Build history of the part. All positions in model axes, mm. A direction names the side the tool comes from. Round coordinates to 2 decimals unless told otherwise and drop trailing zeros. Loops run counter-clockwise (first coordinate to the right, second up) from the corner with the lowest first, then second, coordinate; pieces in that order, holes last. Notation, with made-up numbers: (-17.5, 88.25) - (5.5, 88.25) arc R28 cw to (5.5, 127.25) - close; hole circle Ø1 at (-16.75, 66). An arc over 180 degrees is marked (long way). Put each result on its own line as item: value. Start each with the question number.
Autodesk Inventor part; units mm, degrees
ref_plane "YZ Plane" through (0, 0, 0) normal (1, 0, 0) x (0, 1, 0)
ref_plane "XZ Plane" through (0, 0, 0) normal (0, 1, 0) x (-1, 0, 0)
ref_plane "XY Plane" through (0, 0, 0) normal (0, 0, 1) x (1, 0, 0)
sketch "Sketch1" plane through (0, 0, 0) normal (0, 0, 1) x (1, 0, 0)
  circle A0 centre (0, 0) radius 47.625
  dimension "d0" = 95.25
extrude "Extrusion1" add sketch "Sketch1" along normal blind 3.175
sketch "Sketch3" plane through (0, 0, 3.175) normal (0, 0, 1) x (1, 0, 0)
  line L0 (1.27, 9.525) -> (20.32, 9.525)
  line L1 (20.32, 9.525) -> (20.32, 0)
  line L2 (20.32, 0) -> (1.27, 0)
  line L3 (1.27, 0) -> (1.27, 9.525)
  line L4 (0, 0) -> (0, -11.0035)
  line L5 (-1.27, 9.525) -> (-20.32, 9.525)
  line L6 (-20.32, 9.525) -> (-20.32, 0)
  line L7 (-20.32, 0) -> (-1.27, 0)
  line L8 (-1.27, 0) -> (-1.27, 9.525)
  dimension "d11" = 19.05
  dimension "d12" = 9.525
  dimension "d13" = 1.27
  dimension "d14" = 0
extrude "Extrusion3" add sketch "Sketch3" along normal blind 19.05
sketch "Sketch4" plane through (1.27, 9.525, 3.175) normal (0, 1, 0) x (1, 0, 0)
  circle A0 centre (4.445, -15.24) radius 1.27
  line L0 (19.05, -19.05) -> (0, -19.05)
  circle A1 centre (14.605, -15.24) radius 1.27
  line L1 (9.525, -19.05) -> (9.525, -7.9119)
  line L2 (-1.27, 3.175) -> (-1.27, 8.3959)
  circle A2 centre (-6.985, -15.24) radius 1.27
  circle A3 centre (-17.145, -15.24) radius 1.27
  dimension "d17" = 2.54
  dimension "d18" = 3.81
  dimension "d19" = 2.54
  dimension "d20" = 3.81
  dimension "d21" = 10.16
  dimension "d22" = 5.08
extrude "Extrusion4" cut sketch "Sketch4" against normal through all
sketch "Sketch5" plane through (0, 0, 0) normal (0, 0, -1) x (-1, 0, 0)
  circle A0 centre (10.541, -29.7561) radius 3.25
  point P0 (0, 0)
  dimension "d25" = 6.5
  dimension "d26" = 10.541
  dimension "d27" = 29.7561
extrude "Extrusion5" cut sketch "Sketch5" against normal blind 25.4
sketch "Sketch6" plane through (0, 0, 3.175) normal (0, 0, 1) x (1, 0, 0)
  circle A0 centre (-10.541, -29.7561) radius 3.25
  circle A1 centre (0, 0) radius 47.625
  circle A2 centre (-10.541, -29.7561) radius 9.525
  dimension "d30" = 19.05
extrude "Extrusion6" add sketch "Sketch6" along normal blind 1.27 contours A2
sketch "Sketch7" plane through (0, 0, 0) normal (0, 0, -1) x (-1, 0, 0)
  circle A0 centre (10.541, -29.7561) radius 3.25
  circle A1 centre (0, 0) radius 47.625
  line L0 (5.2005, -29.7561) -> (7.8708, -25.1311)
  line L1 (7.8708, -25.1311) -> (13.2112, -25.1311)
  line L2 (13.2112, -25.1311) -> (15.8815, -29.7561)
  line L3 (15.8815, -29.7561) -> (13.2112, -34.3811)
  line L4 (13.2112, -34.3811) -> (7.8708, -34.3811)
  line L5 (7.8708, -34.3811) -> (5.2005, -29.7561)
  dimension "d33" = 9.25
extrude "Extrusion7" cut sketch "Sketch7" against normal blind 2.54 contours L0 L1 L2 L3 L4 L5
sketch "Sketch8" plane through (0, 0, 3.175) normal (0, 0, 1) x (1, 0, 0)
  line L0 (0, 0) -> (0, 41.91)
  circle A0 centre (0, 41.91) radius 1.5875
  circle A1 centre (-36.2951, 20.955) radius 1.5875
  circle A2 centre (-36.2951, -20.955) radius 1.5875
  circle A3 centre (0, -41.91) radius 1.5875
  circle A4 centre (36.2951, -20.955) radius 1.5875
  circle A5 centre (36.2951, 20.955) radius 1.5875
  dimension "d36" = 41.91
  dimension "d37" = 3.175
  dimension "d40" = 360
extrude "Extrusion8" cut sketch "Sketch8" against normal blind 25.4
properties part number "frontServoAttachmentPlate" material "ABS Plastic"
1) Drill centre lines: line 1 (X direction, y = 20, z = 1.5); line 2 (X direction, y = 6.5, z = 5.75); line 3 (Z direction, x = 5.5, y = 41) (3 decimals). Where is each one in solid material? Low to high. Write a range as [from, to].
2) Slice it at A-A, the plane z = 9.25. Write the cut outline in (x, y) (3 decimals).
3) Drop flat-ended pins along their axis: pin 1 Ø4 at (x, y) = (-37, -16.5) entering from +Z (3 decimals); pin 2 Ø2 at (x, z) = (-11.5, 2) entering from -Y; pin 3 Ø9.5 at (x, y) = (-15, -30) entering from +Z (3 decimals). Give the stop position or say it passes through.
4) Slice it at D-D, the plane y = -9. Write the cut outline in (x, z) (3 decimals), and give its area (3 significant figures).
5) Which spindle directions (+Z, -Z, +X, -X, +Y, -Y) get a long thin tool onto all of the face, cutting with end or side? Do faces 1 (the face through (-11, 9.525, 13)), 2 (the face through (5.44, 4.829, 19.655)), 3 (the face through (-37.555, 19.989, 1.61)), 4 (the face through (-11, -25.131, 1)), 5 (the face through (11, 0, 13)). Say none if no direction does.
6) Slice it at C-C, the plane x = 19. Write the cut outline in (y, z) (3 decimals), and give its area (3 significant figures).
7) Pull direction Y, two halves, no side cores. Call faces 6 (the face through (-37.794, 28.979, 1.565)), 7 (the face through (-20.32, 5, 13)), 8 (the face through (-0.34, 40.36, 1.61)): pulls with the +Y half, pulls with the -Y half, needs draft (parallel to the pull), parting line crosses it, or undercut.
8) Slice it at B-B, the plane y = 41.91. Write the cut outline in (x, z) (1 decimal), and give its area (3 significant figures).
Taken from the geometry:
1. line 1: x = [-43.22, -37.56], [-35.03, 35.03], [37.56, 43.22]
1. line 2: x = [-20.32, -1.27], [1.27, 20.32]
1. line 3: z = [0, 3.175]
2. outline: (-20.32, 0) - (-1.27, 0) - (-1.27, 9.525) - (-20.32, 9.525) - close; (1.27, 0) - (20.32, 0) - (20.32, 9.525) - (1.27, 9.525) - close
3. pin 1: stops at z = 3.175
3. pin 2: stops at y = -46.45
3. pin 3: stops at z = 4.445
4. outline: (-46.767, 0) - (46.767, 0) - (46.767, 3.175) - (-46.767, 3.175) - close
4. area: 297 mm2
5. face 1: +Z, +X, -X, +Y
5. face 2: +Y, -Y
5. face 3: +Z, -Z
5. face 4: -Z
5. face 5: +Z, +X, -X, -Y
6. outline: (-43.671, 0) - (43.671, 0) - (43.671, 3.175) - (9.525, 3.175) - (9.525, 22.225) - (0, 22.225) - (0, 3.175) - (-43.671, 3.175) - close
6. area: 459 mm2
7. face 6: parting line crosses it
7. face 7: needs draft
7. face 8: undercut
8. outline: (-22.6, 0) - (-1.6, 0) - (-1.6, 3.2) - (-22.6, 3.2) - close; (1.6, 0) - (22.6, 0) - (22.6, 3.2) - (1.6, 3.2) - close
8. area: 134 mm2
